Here's how the part is built. I have some questions about the finished solid (model axes, mm). A direction names the side the tool comes from. Coordinates: 2 decimals unless noted, no trailing zeros. Loops run counter-clockwise (first coordinate to the right, second up) from the corner with the lowest first, then second, coordinate; pieces in that order, holes last. Notation, with made-up numbers: (-26.75, 48.5) - (31.25, 48.5) arc R22 cw to (31.25, 65.5) - close; hole circle Ø7 at (61, 57). An arc over 180 degrees is marked (long way). Use a Markdown table: item, result.
```python
from build123d import *

# Parameters (mm, degrees)
ESTRUSIONE_ESTRUSIONE1_DEPTH   = 5
ESTRUSIONE_ESTRUSIONE1_2_DEPTH = 5
SCHIZZO1_3_R                   = 17.5
ESTRUSIONE_ESTRUSIONE2_DEPTH   = 15
FORO_5_0_5_1_D                 = 5


with BuildPart() as part:
    # Schizzo1 → Estrusione-Estrusione1 (new, symmetric)
    with BuildSketch(Plane.XY):
        with BuildLine():
            ThreePointArc((-19.439551712, 41.966109335), (-32.041033104, 47.97699794), (-45.722431864, 45.193575035))
            Line((-45.722431864, 45.193575035), (-40.722431864, 36.533320997))
            ThreePointArc((-40.722431864, 36.533320997), (-20.917414575, 26.550556749), (-16.843225773, 4.749288954))
            ThreePointArc((-16.843225773, 4.749288954), (-6.591441138, 16.211196863), (8.74999975, 15.155444711))
            ThreePointArc((8.74999975, 15.155444711), (7.731749731, 15.829418888), (6.803236294, 16.62247443))
            Line((6.803236294, 16.62247443), (-19.439551712, 41.966109335))
        make_face()
    extrude(amount=ESTRUSIONE_ESTRUSIONE1_DEPTH, both=True)



with BuildPart() as body_2:
    # Schizzo1 → Estrusione-Estrusione1 2 (new, symmetric)
    with BuildSketch(Plane.XY):
        with BuildLine():
            ThreePointArc((17.5, 0), (15.172291449, -8.720755253), (8.808391751, -15.121581755))
            ThreePointArc((8.808391751, -15.121581755), (30.679829856, -9.722971831), (52, -17))
            Line((52, -17), (62, -17))
            ThreePointArc((62, -17), (57.569815566, -3.759849662), (46.063492638, 4.147909046))
            Line((46.063492638, 4.147909046), (10.993866983, 14.203012674))
            ThreePointArc((10.993866983, 14.203012674), (9.842803753, 14.61060124), (8.74999975, 15.155444711))
            ThreePointArc((8.74999975, 15.155444711), (15.155444494, 8.750000125), (17.5, 0))
        make_face()
    extrude(amount=ESTRUSIONE_ESTRUSIONE1_2_DEPTH, both=True)


with BuildPart() as part_1:
    add(part.part)

    add(body_2.part)  # Estrusione-Estrusione2 merges body 2
    # Schizzo1<3> → Estrusione-Estrusione2 (add, symmetric)
    with BuildSketch(Plane.XY):
        Circle(SCHIZZO1_3_R)
        with BuildLine():
            ThreePointArc((2.5, -10.712142643), (0, 11), (-2.5, -10.712142643))
            Line((-2.5, -10.712142643), (-2.5, -13))
            Line((-2.5, -13), (2.5, -13))
            Line((2.5, -13), (2.5, -10.712142643))
        make_face(mode=Mode.SUBTRACT)
    extrude(amount=ESTRUSIONE_ESTRUSIONE2_DEPTH, both=True)

    # Foro Ø5.0 (5)-1 (through all)
    with Locations(Plane.XY.offset(5)):
        with Locations((-38.892304845, 43.363448016), (57, -12)):
            Hole(FORO_5_0_5_1_D / 2)


solid = part_1.part
```
Q1. If we mould it in two halves opening along X, with no side actions, what happens to faces 1 (the face through (-43.257, 40.924, 0.07)), 2 (the face through (54.69, -12.96, -0.07)), 3 (the face through (8, 8, -15))? For each: pulls with the +X half, pulls with the -X half, needs draft (parallel to the pull), parting line crosses it, or undercut.
Check values:
| item | result |
|---|---|
| face 1 | pulls with the -X half |
| face 2 | undercut |
| face 3 | needs draft |
Q2. I want a section at B-B, the plane y = 6. Write out the boundary of the cut face in (x, z).
Check values:
| item | result |
|---|---|
| outline | (-16.53, -5) - (-16.44, -5) - (-16.44, -15) - (-9.22, -15) - (-9.22, 15) - (-16.44, 15) - (-16.44, 5) - (-16.53, 5) - close; (9.22, -15) - (16.44, -15) - (16.44, -5) - (39.6, -5) - (39.6, 5) - (16.44, 5) - (16.44, 15) - (9.22, 15) - close |
Q3. Which directions (+Z, -Z, +X, -X, +Y, -Y) give clear straight access to the entire face, cutting with the end or side of a thin tool? Please do faces 4 (the face through (8, 8, 15)), 5 (the face through (-3.794, -17.084, 0.21)), 6 (the face through (57, -17, 0)).
Check values:
| item | result |
|---|---|
| face 4 | +Z, +X, -X, +Y, -Y |
| face 5 | none |
| face 6 | +Z, -Z, +X, -Y |
Q4. I want a section at A-A, the plane z = 11.5. Write out the boundary of the cut face in (x, y).
Check values:
| item | result |
|---|---|
| outline | circle Ø35 at (0, 0); hole (-2.5, -13) - (2.5, -13) - (2.5, -10.71) arc R11 ccw (long way) to (-2.5, -10.71) - close |
Q5. Please list where these lines run through material, in increasing order: L1, parallel to Y at x = 0, z = 7; L2, parallel to X at y = -8, z = 7; L3, parallel to Y at x = 7, z = -9.5. Write a range as from..to.
Check values:
| item | result |
|---|---|
| L1 | -17.5..-13, 11..17.5 |
| L2 | -15.56..-7.55, 7.55..15.56 |
| L3 | -16.04..-8.49, 8.49..16.04 |
Q6. I want a section at D-D, the plane y = -2.5. Write out the boundary of the cut face in (x, z), then the cut area to 3 significant figures.
Check values:
| item | result |
|---|---|
| outline | (-17.32, -15) - (-10.71, -15) - (-10.71, 15) - (-17.32, 15) - close; (10.71, -15) - (17.32, -15) - (17.32, -5) - (56.55, -5) - (56.55, 5) - (17.32, 5) - (17.32, 15) - (10.71, 15) - close |
| area | 789 mm^2 |
Q7. I want a section at C-C, the plane x = 0. Write out the boundary of the cut face in (y, z), then the cut area to 3 significant figures.
Check values:
| item | result |
|---|---|
| outline | (-17.5, -15) - (-13, -15) - (-13, 15) - (-17.5, 15) - close; (11, -15) - (17.5, -15) - (17.5, -5) - (23.19, -5) - (23.19, 5) - (17.5, 5) - (17.5, 15) - (11, 15) - close |
| area | 387 mm^2 |
Q8. Will these pins go through, and if not, where does the flat tip stop? P1, Ø6, axis at x = -25.5, z = -1.5, coming from the +Y side; P2, Ø3, axis at y = -1, z = -4, coming from the +X side; P3, Ø1.5, axis at y = 24.5, z = 1.5, coming from the +X side; P4, Ø4, axis at x = 57, y = -12, coming from the -Z side.
Check values:
| item | result |
|---|---|
| P1 | y = 47.24 |
| P2 | x = 56.55 |
| P3 | x = -0.58 |
| P4 | through |
